Part model, mm, in its own coordinate system. A direction names the side the tool comes from. Round coordinates to 2 decimals unless told otherwise and drop trailing zeros. Write each loop counter-clockwise with the first axis right and the second up, starting at its lowest first coordinate (ties: lowest second). Pieces come first, ordered by that corner, then holes. Notation, with made-up numbers: (4, 70) -> (11, 70) arc R20 cw to (11, 84) -> close; hole circle Ø9 at (79.5, 70). An arc over 180 degrees is marked (long way). Use CSV: the item, a comma, the result in double quotes. Start each with the question number.
(1) Saw through at C-C (z = 4). Give the cut face in (x, y) (3 decimals), plus the area to 3 significant figures.
(2) Two-plate mould, pull along X, no slides. Class faces 1 (the flat face through (-1, 63.5, 0)), 2 (the flat face through (60.325, 0, 41)), 3 (the flat face through (22.225, 17, 18)): released by +X, released by -X, zero draft, split by the parting line, or undercut.
(3) Saw through at A-A (y = -23). Give the cut face in (x, z) (3 decimals).
(4) Drop flat-ended pins along their axis: pin 1 (5 mm diameter, centred on x = 2.5, z = 20.5, fed in from +Y); pin 2 (17 mm diameter, centred on x = 49.5, z = 51.5, fed in from -Y); pin 3 (6 mm diameter, centred on x = 44, z = 17.5, fed in from +Y); pin 4 (8 mm diameter, centred on x = 43.5, z = 2.5, fed in from +Y). Give the stop position or say it passes through.
(5) Probe line 1 (Z direction, x = -12.5, y = -18.5) (3 decimals); line 2 (Y direction, x = 104.5, z = 43); line 3 (X direction, y = 7, z = 5.5) (3 decimals). List the from-to ranges inside material, lowest first. Write a range as [from, to].
(6) Saw through at B-B (x = 101.5). Give the cut face in (y, z) (3 decimals), plus the area to 3 significant figures.
(7) Which spindle directions (+Z, -Z, +X, -X, +Y, -Y) get a long thin tool onto all of the face, cutting with end or side? Do faces 4 (the flat face through (66, -25.4, 45)), 5 (the cylindrical face through (32.73, -16.79, 51.97)), 6 (the flat face through (66, 25.4, 45)), 7 (the flat face through (-41.275, -1, 0)), 8 (the flat face through (85, 0, 38.1)). Say none if no direction does.
```python
from build123d import *

# Parameters (mm, degrees)
F1_DEPTH = 63.5
F2_DEPTH = 25.4
F3_DEPTH = 7.9375


with BuildPart() as f1:
    # F0 (on Front) → F1 (new body, symmetric)
    with BuildSketch(Plane.XZ):
        Polygon((-41.275, -9.525), (41.275, -9.525), (41.275, 9.525), (22.225, 9.525), (-41.275, 9.525), align=None)
    extrude(amount=F1_DEPTH, both=True)

    # F0 (on Front) → F2 (join, symmetric)
    with BuildSketch(Plane.XZ):
        with BuildLine():
            Line((22.225, 9.525), (41.275, 9.525))
            Line((41.275, 9.525), (41.275, 27.0002))
            ThreePointArc((41.275, 27.0002), (45.92468, 38.22552), (57.15, 42.8752))
            Line((57.15, 42.8752), (60.325, 42.8752))
            Line((60.325, 42.8752), (60.325, 61.9252))
            Line((60.325, 61.9252), (57.15, 61.9252))
            ThreePointArc((57.15, 61.9252), (32.454296, 51.695904), (22.225, 27.0002))
            Line((22.225, 27.0002), (22.225, 9.525))
        make_face()
        Polygon((91.891411, 61.9252), (60.325, 61.9252), (60.325, 42.8752), (74.520705, 42.8752), (91.891411, 42.8752), align=None)
        Polygon((60.325, 66.675), (60.325, 61.9252), (91.891411, 61.9252), (91.891411, 42.8752), (74.520705, 42.8752), (60.325, 42.8752), (60.325, 38.1), (111.125, 38.1), (111.125, 66.675), align=None)
    extrude(amount=F2_DEPTH, both=True)

    # F0 (on Front) → F3 (join, symmetric)
    with BuildSketch(Plane.XZ):
        with BuildLine():
            add(Edge.make_bspline(
                [(-41.275, 9.525), (-28.410731, 53.163726), (38.786519, 65.535851), (57.15, 61.9252)],
                knots=[0, 0, 0, 0, 111.504536, 111.504536, 111.504536, 111.504536], degree=3))
            Line((-41.275, 9.525), (22.225, 9.525))
            Line((22.225, 9.525), (22.225, 27.0002))
            ThreePointArc((22.225, 27.0002), (32.454296, 51.695904), (57.15, 61.9252))
        make_face()
    extrude(amount=F3_DEPTH, both=True)


solid = f1.part
```
Answers:
1,outline,"(-41.275, -63.5) -> (41.275, -63.5) -> (41.275, 63.5) -> (-41.275, 63.5) -> close"
1,area,"10,500 mm²"
2,face 1,"zero draft"
2,face 2,"undercut"
2,face 3,"released by -X"
3,outline,"(-41.275, -9.525) -> (41.275, -9.525) -> (41.275, 27) arc R15.875 cw to (57.15, 42.875) -> (60.325, 42.875) -> (60.325, 38.1) -> (111.125, 38.1) -> (111.125, 66.675) -> (60.325, 66.675) -> (60.325, 61.925) -> (57.15, 61.925) arc R34.925 ccw to (22.225, 27) -> (22.225, 9.525) -> (-41.275, 9.525) -> close"
4,pin 1,"stops at y = 7.94"
4,pin 2,"stops at y = -25.4"
4,pin 3,"stops at y = 25.4"
4,pin 4,"stops at y = 63.5"
5,line 1,"z = [-9.525, 9.525]"
5,line 2,"y = [-25.4, 25.4]"
5,line 3,"x = [-41.275, 41.275]"
6,outline,"(-25.4, 38.1) -> (25.4, 38.1) -> (25.4, 66.675) -> (-25.4, 66.675) -> close"
6,area,"1,450 mm²"
7,face 4,"+Z, +X, -X, -Y"
7,face 5,"+Z, -X, -Y"
7,face 6,"+Z, +X, -X, +Y"
7,face 7,"+Z, -Z, -X, +Y, -Y"
7,face 8,"-Z, +X, +Y, -Y"
